```python
from build123d import *

# Parameters (mm, degrees)
F0_R     = 25
F1_DEPTH = 24
F2_R     = 12
F3_DEPTH = 6
F4_R     = 6
F5_DEPTH = 30.001


with BuildPart() as f1:
    # F0 (on Front) → F1 (new body)
    with BuildSketch(Plane.XZ):
        Circle(F0_R)
    extrude(amount=F1_DEPTH)

    # F2 (on face) → F3 (join)
    with BuildSketch(Plane.XZ.offset(24)):
        Circle(F2_R)
    extrude(amount=F3_DEPTH)

    # F4 (on face) → F5 (cut, through all)
    with BuildSketch(Plane(origin=(0, 0, 0), x_dir=(-1, 0, 0), z_dir=(0, 1, 0))):
        Circle(F4_R)
    extrude(amount=-F5_DEPTH, mode=Mode.SUBTRACT)


solid = f1.part
```
Build history of the part. All positions in model axes, mm. A direction names the side the tool comes from. Give positions to 0.01 mm unless a question says otherwise; leave off trailing zeros. Loops run counter-clockwise (first coordinate to the right, second up) from the corner with the lowest first, then second, coordinate; pieces in that order, holes last. Notation, with made-up numbers: (-11, 41.25) -> (24, 41.25) arc R20 cw to (24, 63.25) -> close; hole circle Ø10 at (-18, -28). An arc over 180 degrees is marked (long way). One line per question, with ' | ' between items.
Q1. Cut at B-B, the plane z = 0. Write the cut outline in (x, y), plus the area to 3 significant figures.
Filled sheet:
outline: (-25, -24) -> (-12, -24) -> (-12, -30) -> (-6, -30) -> (-6, 0) -> (-25, 0) -> close; (6, -30) -> (12, -30) -> (12, -24) -> (25, -24) -> (25, 0) -> (6, 0) -> close | area: 984 mm²
Q2. Cut at A-A, the plane x = 0. Write the cut outline in (y, z), plus the area to 3 significant figures.
Filled sheet:
outline: (-30, -12) -> (-24, -12) -> (-24, -25) -> (0, -25) -> (0, -6) -> (-30, -6) -> close; (-30, 6) -> (0, 6) -> (0, 25) -> (-24, 25) -> (-24, 12) -> (-30, 12) -> close | area: 984 mm²
Q3. Cut at D-D, the plane z = 13. Write the cut outline in (x, y).
Filled sheet:
outline: (-21.35, -24) -> (21.35, -24) -> (21.35, 0) -> (-21.35, 0) -> close
Q4. Tool access for faces 1 (the cylindrical face through (-11.99, -26.96, 0.53)), 2 (the cylindrical face through (23.846, -11.832, 7.509)): list every direction of +Z, -Z, +X, -X, +Y, -Y with a clear straight run to the whole face (end or side of a thin tool).
Filled sheet:
face 1: -Y | face 2: +Y, -Y
Q5. Cut at C-C, the plane y = -16.25. Write the cut outline in (x, z).
Filled sheet:
outline: circle Ø50 at (0, 0); hole circle Ø12 at (0, 0)
Q6. Drop flat-ended pins along their axis: pin 1 (1.5 mm diameter, centred on y = -22.5, z = -15.5, fed in from -X); pin 2 (10 mm diameter, centred on x = 15.5, y = -23, fed in from +Z); pin 3 (1.5 mm diameter, centred on y = -21.5, z = -2, fed in from -X). Give the stop position or say it passes through.
Filled sheet:
pin 1: stops at x = -20.19 | pin 2: stops at z = 22.69 | pin 3: stops at x = -24.97
Q7. Drill centre lines: line 1 along Z through (x, y) = (0, -22.25); line 2 along Y through (x, z) = (14.5, -1); line 3 along X through (y, z) = (-20.5, 2). Where is each one in solid material? Low to high. Write a range as [from, to].
Filled sheet:
line 1: z = [-25, -6], [6, 25] | line 2: y = [-24, 0] | line 3: x = [-24.92, -5.66], [5.66, 24.92]
